Design review of the part built by this model. Coordinates are the model's own, in mm. A direction names the side the tool comes from. Give positions to 0.01 mm unless a question says otherwise; leave off trailing zeros. Write each loop counter-clockwise with the first axis right and the second up, starting at its lowest first coordinate (ties: lowest second). Pieces come first, ordered by that corner, then holes. Notation, with made-up numbers: M 12,47 L 34,47 A9 ccw 34,52 Z; hole C 52.25,11 d7. An arc over 180 degrees is marked long. Use a Markdown table: item, result. Add a question column.
Autodesk Inventor part; units mm, degrees
ref_plane "YZ Plane" through (0, 0, 0) normal (1, 0, 0) x (0, 1, 0)
ref_plane "XZ Plane" through (0, 0, 0) normal (0, 1, 0) x (-1, 0, 0)
ref_plane "XY Plane" through (0, 0, 0) normal (0, 0, 1) x (1, 0, 0)
sketch "Sketch1" plane through (0, 0, 0) normal (0, 1, 0) x (-1, 0, 0)
  circle A0 centre (0, 0) radius 2.35
  line L0 (0, 0) -> (0, -22.5)
  circle A1 centre (0, -22.5) radius 1
  circle A2 centre (0, 22.5) radius 1
  circle A3 centre (0, -22.5) radius 2
  circle A4 centre (0, 22.5) radius 2
  circle A5 centre (0, 0) radius 5
  line L1 (5, 0) -> (4.8273, 1.3027)
  line L2 (-5, 0) -> (-4.8273, 1.3027)
  line L3 (-5, 0) -> (-1.9827, -22.7628)
  line L4 (5, 0) -> (1.9827, -22.7628)
  circle A6 centre (0, 0) radius 1
  line L5 (0, 0) -> (0, 5)
  line L6 (0, 20.5) -> (0, 22.5)
  dimension "d6" = 4
  dimension "d0" = 4.7
  dimension "d1" = 22.5
  dimension "d2" = 22.5
  dimension "d3" = 2
  dimension "d4" = 2
  dimension "d5" = 4
  dimension "d7" = 10
  dimension "d8" = 2
extrude "Extrusion3" add sketch "Sketch1" along normal blind 3 contours A0 L0 A6 L5 | A0 L5 A5 L1 L4 L0 | L5 A6 L0 A0 | A0 L0 A5 L3 L2 L5 | A5 L4 A3 L0 | L0 A3 L3 A5 | A3
extrude "Extrusion4" cut sketch "Sketch1" along normal blind 2.5 contours A0 L0 A6 L5 | L5 A6 L0 A0
properties part number "ServoYAxis"
(1) Add section B-B on y = 1.6. Give the boundary of the cut face in (x, z), then the cut area to 3 significant figures.
(2) Machinability: for faces 4 (the cylindrical face through (0.509, 1.232, 2.294)), 5 (the cylindrical face through (0, 1.5, -24.5)), which of the approach directions +Z, -Z, +X, -X, +Y, -Y give a long, thin tool a straight path to every point of the face, cutting with its end or side? Answer none if there is none.
(3) Add section A-A on x = 0. Give the boundary of the cut face in (y, z), then the cut area to 4 significant figures.
(4) For pin 1 (1.2 mm diameter, centred on x = 0, z = 0, fed in from -Y); pin 2 (1.5 mm diameter, centred on y = 2.5, z = -4.5, fed in from -X); pin 3 (1.4 mm diameter, centred on x = 0.5, z = -0.5, fed in from -Y); pin 4 (2.5 mm diameter, centred on x = 0, z = -22.5, fed in from +Y), all flat-tipped, find the tip position at first contact; note any pin that passes through.
(5) Add section D-D on x = -2.75. Give the boundary of the cut face in (y, z), then the cut area to 4 significant figures.
(6) The part is to be moulded in two halves that separate along Z. For faces 1 (the cylindrical face through (0.217, 2.746, 0.976)), 2 (the flat face through (4.915, 1.479, 0.642)), 3 (the flat face through (0, 3, -6)), say which applies: released by +Z, released by -Z, zero draft, split by the parting line, or undercut.
(7) Add section C-C on z = -11.25. Give the boundary of the cut face in (x, y), then the cut area to 3 significant figures.
(8) Wall thickness on L1, parallel to Z at x = 0, y = 1.9; L2, parallel to X at y = 2.6, z = 0; L3, parallel to X at y = 2.25, z = 2: over which ranges is each line inside the solid? List them lowest first.
From the geometry:
| question | item | result |
|---|---|---|
| 1 | outline | M -5,0 L -1.98,-22.76 A2 ccw 1.98,-22.76 L 5,0 L 4.83,1.3 A5 ccw -4.83,1.3 Z; hole C 0,0 d4.7; hole C 0,-22.5 d2 |
| 1 | area | 183 mm^2 |
| 2 | face 4 | -Y |
| 2 | face 5 | -Z, +Y, -Y |
| 3 | outline | M 0,-24.5 L 3,-24.5 L 3,-23.5 L 0,-23.5 Z; M 0,-21.5 L 3,-21.5 L 3,-1 L 2.5,-1 L 2.5,-2.35 L 0,-2.35 Z; M 0,2.35 L 2.5,2.35 L 2.5,1 L 3,1 L 3,5 L 0,5 Z |
| 3 | area | 69.75 mm^2 |
| 4 | pin 1 | passes through |
| 4 | pin 2 | stops at x = -4.5 |
| 4 | pin 3 | stops at y = 2.5 |
| 4 | pin 4 | stops at y = 3 |
| 5 | outline | M 0,-16.97 L 3,-16.97 L 3,4.18 L 0,4.18 Z |
| 5 | area | 63.45 mm^2 |
| 6 | face 1 | undercut |
| 6 | face 2 | released by +Z |
| 6 | face 3 | zero draft |
| 7 | outline | M -3.51,0 L 3.51,0 L 3.51,3 L -3.51,3 Z |
| 7 | area | 21.1 mm^2 |
| 8 | L1 | z = -24.5 to -23.5, -21.5 to -2.35, 2.35 to 5 |
| 8 | L2 | x = -5 to -1, 1 to 5 |
| 8 | L3 | x = -4.58 to -1.23, 1.23 to 4.58 |
